For this review, take the finished solid that the model builds, in its own axes (mm). Coordinates: 2 decimals unless noted, no trailing zeros. Loops run counter-clockwise (first coordinate to the right, second up) from the corner with the lowest first, then second, coordinate; pieces in that order, holes last. Notation, with made-up numbers: M 78,43 L 96,43 A23 ccw 96,77 Z; hole C 51.5,31.25 d1. An arc over 180 degrees is marked long. Answer as a JSON object with one key per item and string values. Group by question number.
Item 1: Add section A-A (x = -4.5). State the section outline as (y, z) points, then the cut area to 3 significant figures.
Item 2: Mouldability with a two-part tool opening along X and no side actions: class faces 1 (the face through (-15, 0, 4)), 2 (the face through (-9.059, -9.274, 4.056)), 3 (the face through (15, 0, 4)), 4 (the face through (0, -15, 4)) as +X half, -X half, draft (parallel to the pull), parting line (faces both ways), or undercut.
Item 3: Add section B-B (y = 10.75). State the section outline as (x, z) points.
Item 4: Add section C-C (y = 0). State the section outline as (x, z) points.
Item 5: Insertion check: pin 1 (5.5 mm diameter, centred on x = 10, y = -10.75, fed in from +Z); pin 2 (3 mm diameter, centred on x = 10, y = 10.75, fed in from -Z). Each pin has a flat end and moves straight along its axis. Give the tip position at first contact, or say it passes through.
Item 6: Add section D-D (x = 10). State the section outline as (y, z) points, then the cut area to 3 significant figures.
Item 7: Wall thickness on L1, parallel to Y at x = -10, z = 4; L2, parallel to X at y = 9.5, z = 1; L3, parallel to Y at x = 0, z = 2.5: over which ranges is each line inside the solid? List them lowest first. Write a range as from..to.
Autodesk Inventor part; units mm, degrees
ref_plane "YZ Plane" through (0, 0, 0) normal (1, 0, 0) x (0, 1, 0)
ref_plane "XZ Plane" through (0, 0, 0) normal (0, 1, 0) x (-1, 0, 0)
ref_plane "XY Plane" through (0, 0, 0) normal (0, 0, 1) x (1, 0, 0)
sketch "Sketch1" plane through (0, 0, 0) normal (0, 0, 1) x (1, 0, 0)
  line L0 (-15, 15) -> (15, 15)
  line L1 (15, 15) -> (15, -15)
  line L2 (15, -15) -> (-15, -15)
  line L3 (-15, -15) -> (-15, 15)
  point P0 (0, 0)
  point P1 (0, 15)
  point P2 (-15, 0)
  dimension "d0" = 30
  dimension "d1" = 30
extrude "Extrusion1" add sketch "Sketch1" along normal blind 8
sketch "Sketch2" plane through (0, 0, 8) normal (0, 0, 1) x (1, 0, 0)
  circle A0 centre (0, 0) radius 7.5
  line L0 (15, 15) -> (-15, 15)
  line L1 (-15, 15) -> (-15, -15)
  point P0 (0, 15)
  point P1 (-15, 0)
  dimension "d17" = 15
extrude "Extrusion2" cut sketch "Sketch2" against normal through all
sketch "Sketch3" plane through (0, 0, 8) normal (0, 0, 1) x (1, 0, 0)
  circle A0 centre (10, -10.75) radius 1.75
  circle A1 centre (10, 10.75) radius 1.75
  line L0 (15, 15) -> (-15, 15)
  line L1 (15, -15) -> (15, 15)
  circle A2 centre (-10, -10.75) radius 1.75
  circle A3 centre (-10, 10.75) radius 1.75
  line L2 (-15, 15) -> (-15, -15)
  line L3 (-15, -15) -> (15, -15)
  line L4 (10, 10.75) -> (-10, 10.75) construction
  line L5 (-10, 10.75) -> (-10, -10.75) construction
  line L6 (-10, -10.75) -> (10, -10.75) construction
  line L7 (10, -10.75) -> (10, 10.75) construction
  point P0 (0, 0)
  point P1 (10, 0)
  point P2 (0, 10.75)
  dimension "d9" = 3.5
  dimension "d19" = 10.75
  dimension "d20" = 10.75
  dimension "d21" = 20
  dimension "d22" = 21.5
extrude "Extrusion3" cut sketch "Sketch3" against normal through all contours A0 | A1 | A2 | A3
properties part number "0005-10-006 Capac rulment"
From the geometry:
{
 "1": {"outline": "M -15,0 L -6,0 L -6,8 L -15,8 Z; M 6,0 L 15,0 L 15,8 L 6,8 Z", "area": "144 mm²"},
 "2": {"face 1": "-X half", "face 2": "undercut", "face 3": "+X half", "face 4": "draft"},
 "3": {"outline": "M -15,0 L -11.75,0 L -11.75,8 L -15,8 Z; M -8.25,0 L 8.25,0 L 8.25,8 L -8.25,8 Z; M 11.75,0 L 15,0 L 15,8 L 11.75,8 Z"},
 "4": {"outline": "M -15,0 L -7.5,0 L -7.5,8 L -15,8 Z; M 7.5,0 L 15,0 L 15,8 L 7.5,8 Z"},
 "5": {"pin 1": "stops at z = 8", "pin 2": "passes through"},
 "6": {"outline": "M -15,0 L -12.5,0 L -12.5,8 L -15,8 Z; M -9,0 L 9,0 L 9,8 L -9,8 Z; M 12.5,0 L 15,0 L 15,8 L 12.5,8 Z", "area": "184 mm²"},
 "7": {"L1": "y = -15..-12.5, -9..9, 12.5..15", "L2": "x = -15..-11.22, -8.78..8.78, 11.22..15", "L3": "y = -15..-7.5, 7.5..15"}
}
